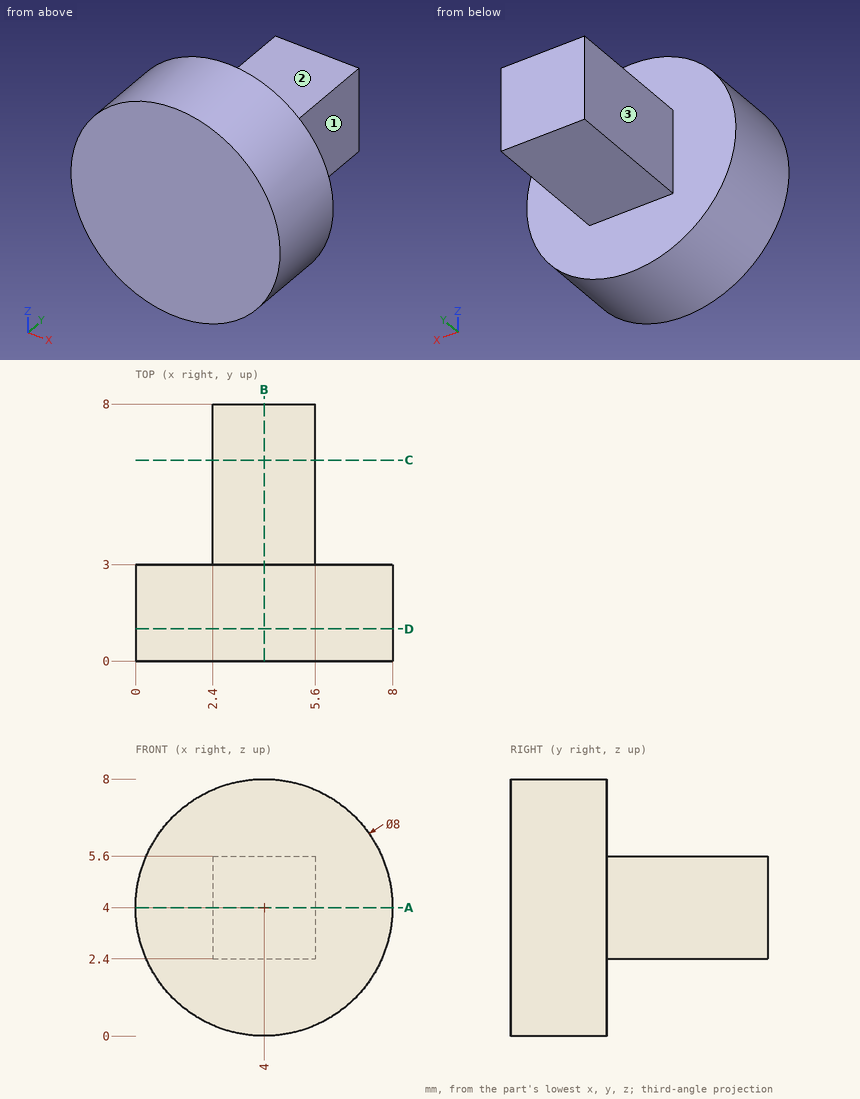
Part print with two shaded views. Sizes in mm from the minimum x, y, z corner. A direction names the side the tool comes from. Give positions to 0.01 mm unless a question says otherwise; leave off trailing zeros. Order: outer loops, then holes, each group sorted by start corner. A loop starts at its lowest first (then second) coordinate and runs counter-clockwise, first axis right, second up. Notation, with made-up numbers: M -21,-28.75 L -15,-28.75 A16 ccw -15,-1.75 Z; hole C 37.5,76 d11. An arc over 180 degrees is marked long. Put each result on its own line as item: value.
Item 1: Cut at A-A on z = 4. Write the cut outline in (x, y).
Results are:
outline: M 0,0 L 8,0 L 8,3 L 5.6,3 L 5.6,8 L 2.4,8 L 2.4,3 L 0,3 Z
Item 2: Which spindle directions (+Z, -Z, +X, -X, +Y, -Y) get a long thin tool onto all of the face, cutting with end or side? Do the marked faces 1, 2 and 3. Say none if no direction does.
Results are:
face 1: +Z, -Z, +X, +Y
face 2: +Z, +X, -X, +Y
face 3: +Z, -Z, -X, +Y
Item 3: Cut at D-D on y = 1. Write the cut outline in (x, z), then the cut area to 3 significant figures.
Results are:
outline: C 4,4 d8
area: 50.3 mm2
Item 4: Drop flat-ended pins along their axis: pin 1 Ø1 at (y, z) = (2.5, 1.5) entering from -X; pin 2 Ø3 at (x, z) = (1, 6.5) entering from +Y; pin 3 Ø1.6 at (y, z) = (6.5, 3.5) entering from -X. Give the stop position or say it passes through.
Results are:
pin 1: x = 0.54
pin 2: y = 3
pin 3: x = 2.4
Item 5: Wall check: probe 1 along Y at (x, z) = (7.25, 4.25); probe 2 along Z at (x, y) = (2.75, 4.75). Give the ranges that are in metal, low to high.
Results are:
probe 1: 0 to 3
probe 2: 2.4 to 5.6
Item 6: Cut at B-B on x = 4. Write the cut outline in (y, z), then the cut area to 3 significant figures.
Results are:
outline: M 0,0 L 3,0 L 3,2.4 L 8,2.4 L 8,5.6 L 3,5.6 L 3,8 L 0,8 Z
area: 40.0 mm2
Item 7: Cut at C-C on y = 6.25. Write the cut outline in (x, z).
Results are:
outline: M 2.4,2.4 L 5.6,2.4 L 5.6,5.6 L 2.4,5.6 Z
